from build123d import *

# Parameters (mm, degrees)
CUT_EXTRUDE_1_DEPTH = 40


with BuildPart() as part:
    # 草图1 → 旋转1 (revolve)
    with BuildSketch(Plane(origin=(0, 0, 0), x_dir=(0, 0, -1), z_dir=(1, 0, 0)), mode=Mode.PRIVATE) as revolve_1_sk:
        with BuildLine():
            Line((0, 15.3), (0, 16.196152423))
            ThreePointArc((0, 16.196152423), (0.102222521, 16.972609558), (0.401923789, 17.696152423))
            Line((0.401923789, 17.696152423), (4.440192379, 24.690638796))
            ThreePointArc((4.440192379, 24.690638796), (4.777645714, 24.830416543), (5, 24.540638796))
            Line((5, 24.540638796), (5, 18))
            Line((5, 18), (55, 18))
            Line((55, 18), (55, 15))
            Line((55, 15), (2.5, 15))
            Line((2.5, 15), (2.5, 16))
            Line((2.5, 16), (1, 16))
            Line((1, 16), (1, 15))
            Line((1, 15), (0.3, 15))
            ThreePointArc((0.3, 15), (0.087867966, 15.087867966), (0, 15.3))
        make_face()
    revolve(revolve_1_sk.sketch.rotate(Axis((0, 0, 31.844262295), (0, 0, -1)), 90), axis=Axis((0, 0, 31.844262295), (0, 0, -1)))

    # 草图2 → 切除-拉伸1 (cut)
    with BuildSketch(Plane(origin=(0, 0, -55), x_dir=(-1, 0, 0), z_dir=(0, 0, -1))):
        with BuildLine():
            Line((-5, 17.291616466), (-5, 15.198684154))
            ThreePointArc((-5, 15.198684154), (-11.313708499, 11.313708499), (-15.198684154, 5))
            Line((-15.198684154, 5), (-17.291616466, 5))
            ThreePointArc((-17.291616466, 5), (-12.727922061, 12.727922061), (-5, 17.291616466))
        make_face()
        with BuildLine():
            Line((5, 17.291616466), (5, 15.198684154))
            ThreePointArc((5, 15.198684154), (11.313708499, 11.313708499), (15.198684154, 5))
            Line((15.198684154, 5), (17.291616466, 5))
            ThreePointArc((17.291616466, 5), (12.727922061, 12.727922061), (5, 17.291616466))
        make_face()
        with BuildLine():
            Line((-17.291616466, -5), (-15.198684154, -5))
            ThreePointArc((-15.198684154, -5), (-11.313708499, -11.313708499), (-5, -15.198684154))
            Line((-5, -15.198684154), (-5, -17.291616466))
            ThreePointArc((-5, -17.291616466), (-12.727922061, -12.727922061), (-17.291616466, -5))
        make_face()
        with BuildLine():
            Line((15.198684154, -5), (17.291616466, -5))
            ThreePointArc((17.291616466, -5), (12.727922061, -12.727922061), (5, -17.291616466))
            Line((5, -17.291616466), (5, -15.198684154))
            ThreePointArc((5, -15.198684154), (11.313708499, -11.313708499), (15.198684154, -5))
        make_face()
    extrude(amount=-CUT_EXTRUDE_1_DEPTH, mode=Mode.SUBTRACT)


solid = part.part
Source: CAD feature listing. Evaluate the final solid. Frame: model axes, mm. A direction names the side the tool comes from. Round coordinates to 2 decimals unless told otherwise and drop trailing zeros. Loops run counter-clockwise (first coordinate to the right, second up) from the corner with the lowest first, then second, coordinate; pieces in that order, holes last. Notation, with made-up numbers: (17.25, -31) -> (49.25, -31) arc R23 ccw to (49.25, -22) -> close; hole circle Ø4 at (74.5, 72.25). An arc over 180 degrees is marked (long way). Answer as a JSON object with one key per item and string values. Group by question number.
Q1. Section query D-D (z = -6.5). Output: boundary loops of the cut face in (x, y).
Q2. Mould query, pull axis X, two halves, no side actions, for faces 5 (the flat face through (-12, 11, -15)), 6 (the conical face through (-3.931, 17.702, -0.655)), 7 (the cylindrical face through (-3.47, 15.62, -1.74)). Classes: pulls with the +X half, pulls with the -X half, needs draft (parallel to the pull), parting line crosses it, or undercut.
Q3. Section query B-B (x = 0). Output: boundary loops of the cut face in (y, z), plus the area to 3 significant figures.
Q4. Ray query, line 1 (Y direction, x = 0, z = -43); line 2 (Y direction, x = 4, z = -6); line 3 (X direction, y = -11, z = -30). Return the intervals inside material, ascending. Write a range as from..to.
Q5. Section query A-A (z = -47.5). Output: boundary loops of the cut face in (x, y), plus the area to 3 significant figures.
Q6. Contact query for flat-ended pins moving along their axis: P1, Ø2.5, axis at x = 16, z = -37, coming from the -Y side; P2, Ø8, axis at x = 13, z = -19.5, coming from the +Y side; P3, Ø10, axis at y = -18.5, z = -46, coming from the +X side. Output: stop coordinate, or through.
Q7. Access query for faces 1 (the flat face through (-12, -12, -15)), 2 (the flat face through (12, 11, -15)), 3 (the flat face through (-13, -13, -5)), 4 (the flat face through (5, -16, -35)). Directions: +Z, -Z, +X, -X, +Y, -Y. A direction counts if a zero-diameter tool reaches every point of the face in a straight line with its end or side. Return the directions, or none.
Completed:
{
 "1": {"outline": "circle Ø36 at (0, 0); hole circle Ø30 at (0, 0)"},
 "2": {"face 5": "needs draft", "face 6": "parting line crosses it", "face 7": "undercut"},
 "3": {"outline": "(-24.69, -4.44) arc R0.3 ccw to (-24.54, -5) -> (-18, -5) -> (-18, -55) -> (-15, -55) -> (-15, -2.5) -> (-16, -2.5) -> (-16, -1) -> (-15, -1) -> (-15, -0.3) arc R0.3 ccw to (-15.3, 0) -> (-16.2, 0) arc R3 ccw to (-17.7, -0.4) -> close; (15, -55) -> (18, -55) -> (18, -5) -> (24.54, -5) arc R0.3 ccw to (24.69, -4.44) -> (17.7, -0.4) arc R3 ccw to (16.2, 0) -> (15.3, 0) arc R0.3 ccw to (15, -0.3) -> (15, -1) -> (16, -1) -> (16, -2.5) -> (15, -2.5) -> close", "area": "360 mm²"},
 "4": {"line 1": "-18..-15, 15..18", "line 2": "-17.55..-14.46, 14.46..17.55", "line 3": "-11.62..-10.2, 10.2..11.62"},
 "5": {"outline": "(-17.29, -5) -> (-15.2, -5) arc R16 ccw to (-5, -15.2) -> (-5, -17.29) arc R18 ccw to (5, -17.29) -> (5, -15.2) arc R16 ccw to (15.2, -5) -> (17.29, -5) arc R18 ccw to (17.29, 5) -> (15.2, 5) arc R16 ccw to (5, 15.2) -> (5, 17.29) arc R18 ccw to (-5, 17.29) -> (-5, 15.2) arc R16 ccw to (-15.2, 5) -> (-17.29, 5) arc R18 ccw to start; hole circle Ø30 at (0, 0)", "area": "179 mm²"},
 "6": {"P1": "y = -6.2", "P2": "y = 13.23", "P3": "x = 8.59"},
 "7": {"face 1": "-Z, -X, -Y", "face 2": "-Z, +X, +Y", "face 3": "-Z", "face 4": "-Z, +X, -Y"}
}
